```python
from build123d import *

# Parameters (mm, degrees)
SKETCH_1_W                  = 67
SKETCH_1_H                  = 21
EXTRUDE_1_DEPTH             = 45
SHELL_1_T                   = -1
FILLET_1_R                  = 0.5
CHAMFER_1_SIZE              = 5
HOLE_WIZARD_10_0_10_1_D     = 10
HOLE_WIZARD_10_0_10_1_DEPTH = 1
HOLE_WIZARD_10_0_10_2_D     = 10
HOLE_WIZARD_3_5_3_5_1_D     = 3.5


with BuildPart() as part:
    # 草图1 → 凸台-拉伸1 (new body)
    with BuildSketch(Plane(origin=(0, 0, 0), x_dir=(1, 0, 0), z_dir=(0, 1, 0))):
        with Locations((-33.5, 10.5)):
            Rectangle(SKETCH_1_W, SKETCH_1_H)
    extrude(amount=EXTRUDE_1_DEPTH)

    # 抽壳1
    shell_1_openings = [part.faces().sort_by_distance(p)[0] for p in [
        (-33.5, 45, -10.5),
        (-33.5, 22.5, 0),
        (-33.5, 22.5, -21),
    ]]
    offset(amount=SHELL_1_T, openings=shell_1_openings, kind=Kind.INTERSECTION)

    # 圆角1
    fillet_1_edges = [part.edges().sort_by_distance(p)[0] for p in [
        (-67, 0, -10.5),
        (0, 0, -10.5),
    ]]
    fillet(fillet_1_edges, radius=FILLET_1_R)

    # 倒角1
    chamfer_1_edges = [part.edges().sort_by_distance(p)[0] for p in [
        (-66.5, 45, 0),
        (-66.5, 45, -21),
        (-0.5, 45, 0),
        (-0.5, 45, -21),
    ]]
    chamfer(chamfer_1_edges, length=CHAMFER_1_SIZE)

    # Ø10.0 (10) 直径槽口1
    with Locations(Plane.ZY.offset(67)):
        with Locations((-10.5, 35)):
            Hole(HOLE_WIZARD_10_0_10_1_D / 2, depth=HOLE_WIZARD_10_0_10_1_DEPTH)

    # Ø10.0 (10) 直径槽口2 (through all)
    with Locations(Plane(origin=(0, 1, 0), x_dir=(1, 0, 0), z_dir=(0, 1, 0))):
        with Locations((-24.5, 10.5)):
            Hole(HOLE_WIZARD_10_0_10_2_D / 2)

    # Ø3.5 (3.5) 直径槽口1 (through all)
    with Locations(Plane(origin=(0, 0, 0), x_dir=(0, 0, -1), z_dir=(1, 0, 0))):
        with Locations((10.5, 35)):
            Hole(HOLE_WIZARD_3_5_3_5_1_D / 2)


solid = part.part
```
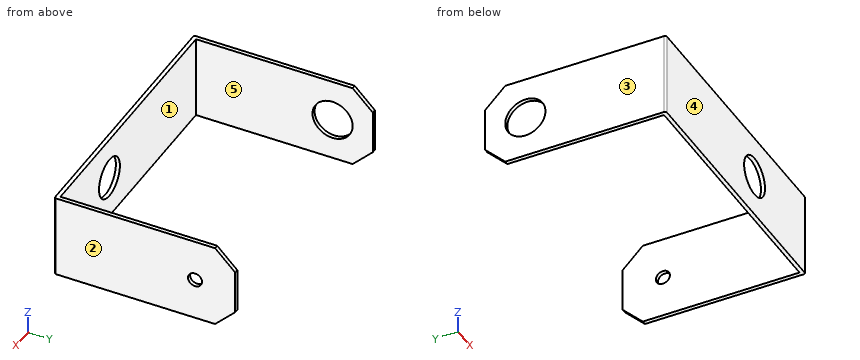
For this review, take the finished solid that the model builds, in its own axes (mm). Face numbers are marked on the shaded views. A direction names the side the tool comes from. Round coordinates to 2 decimals unless told otherwise and drop trailing zeros. Write each loop counter-clockwise with the first axis right and the second up, starting at its lowest first coordinate (ties: lowest second). Pieces come first, ordered by that corner, then holes. Notation, with made-up numbers: M -20,-11.5 L 20,-11.5 A11 cw 20,-6.5 Z; hole C 62.5,-4.75 d5. An arc over 180 degrees is marked long. One line per item, written item: value. Start each with the question number.
(1) The part is to be moulded in two halves that separate along X. For the marked faces 3, 4 and 5, say which applies: released by +X, released by -X, zero draft, split by the parting line, or undercut.
(2) We need section A-A (x = -24.5). Give the boundary of the cut face in (y, z).
(3) Wall thickness on line 1 (X direction, y = 20.5, z = -13.5); line 2 (Z direction, x = -24.5, y = 0.65); line 3 (Y direction, x = -29.5, z = -1.5): over which ranges is each line inside the solid? List them lowest first.
(4) We need section B-B (y = 35). Give the boundary of the cut face in (x, z).
(5) We need section C-C (z = -10.5). Give the boundary of the cut face in (x, y), and give its area (3 significant figures).
(6) Insertion check: pin 1 (6.5 mm diameter, centred on x = -42, z = -11.5, fed in from +Y); pin 2 (10 mm diameter, centred on x = -25, y = 9, fed in from -Z). Each pin has a flat end and moves straight along its axis. Give the tip position at first contact, or say it passes through.
(7) Machinability: for the marked faces 1 and 2, which of the approach directions +Z, -Z, +X, -X, +Y, -Y give a long, thin tool a straight path to every point of the face, cutting with its end or side? Answer none if there is none.
(8) We need section D-D (y = 4.5). Give the boundary of the cut face in (x, z), and give its area (3 significant figures).
Result:
1. face 3: released by -X
1. face 4: zero draft
1. face 5: undercut
2. outline: M 0,-21 L 1,-21 L 1,-15.5 L 0,-15.5 Z; M 0,-5.5 L 1,-5.5 L 1,0 L 0,0 Z
3. line 1: -67 to -66, -1 to 0
3. line 2: -21 to -15.5, -5.5 to 0
3. line 3: 0 to 1
4. outline: M -67,-21 L -66,-21 L -66,-15.5 L -67,-15.5 Z; M -67,-5.5 L -66,-5.5 L -66,0 L -67,0 Z; M -1,-21 L 0,-21 L 0,-12.25 L -1,-12.25 Z; M -1,-8.75 L 0,-8.75 L 0,0 L -1,0 Z
5. outline: M -67,0.5 A0.5 ccw -66.5,0 L -29.5,0 L -29.5,1 L -66,1 L -66,30 L -67,30 Z; M -67,40 L -66,40 L -66,45 L -67,45 Z; M -19.5,0 L -0.5,0 A0.5 ccw 0,0.5 L 0,33.25 L -1,33.25 L -1,1 L -19.5,1 Z; M -1,36.75 L 0,36.75 L 0,45 L -1,45 Z
5. area: 131 mm²
6. pin 1: y = 1
6. pin 2: through
7. face 1: +Z, -Z, +Y
7. face 2: +Z, -Z, +X, +Y, -Y
8. outline: M -67,-21 L -66,-21 L -66,0 L -67,0 Z; M -1,-21 L 0,-21 L 0,0 L -1,0 Z
8. area: 42.0 mm²
